from build123d import *

# Parameters (mm, degrees)
F0_W      = 78
F0_H      = 3
F1_DEPTH  = 78
F2_W      = 4
F2_H      = 78
F3_DEPTH  = 28
F4_W      = 4
F4_H      = 78
F5_DEPTH  = 28
F6_W      = 78
F6_H      = 3
F7_DEPTH  = 15
F8_W      = 78
F8_H      = 3
F9_DEPTH  = 15
F12_R     = 3.217192
F13_DEPTH = 22.5
F14_R     = 3.037913
F15_DEPTH = 18.4
F10_R     = 6.245135
F16_DEPTH = 2
F11_R     = 4
F17_DEPTH = 12.6


with BuildPart() as f1:
    # F0 (on Front) → F1 (new body)
    with BuildSketch(Plane.XZ):
        with Locations((4.030592, -1.5)):
            Rectangle(F0_W, F0_H)
    extrude(amount=F1_DEPTH)

    # F2 (on face) → F3 (join)
    with BuildSketch(Plane.XY):
        with Locations((-32.969408, -39)):
            Rectangle(F2_W, F2_H)
    extrude(amount=F3_DEPTH)

    # F4 (on face) → F5 (join)
    with BuildSketch(Plane.XY):
        with Locations((41.030592, -39)):
            Rectangle(F4_W, F4_H)
    extrude(amount=F5_DEPTH)

    # F6 (on face) → F7 (join)
    with BuildSketch(Plane(origin=(-34.969408, 0, 0), x_dir=(0, -1, 0), z_dir=(-1, 0, 0))):
        with Locations((39, 26.5)):
            Rectangle(F6_W, F6_H)
    extrude(amount=F7_DEPTH)

    # F8 (on face) → F9 (join)
    with BuildSketch(Plane.YZ.offset(43.030592)):
        with Locations((-39, 26.5)):
            Rectangle(F8_W, F8_H)
    extrude(amount=F9_DEPTH)

    # F12 (on face) → F13 (cut)
    with BuildSketch(Plane.XY.offset(28)):
        with Locations((47.882639, -9.369526)):
            Circle(F12_R)
        with Locations((47.882639, -68.630474)):
            Circle(F12_R)
    extrude(amount=-F13_DEPTH, mode=Mode.SUBTRACT)

    # F14 (on face) → F15 (cut)
    with BuildSketch(Plane.XY.offset(28)):
        with Locations((-40.469408, -8.328774)):
            Circle(F14_R)
        with Locations((-40.469408, -69.671226)):
            Circle(F14_R)
    extrude(amount=-F15_DEPTH, mode=Mode.SUBTRACT)

    # F10 (on face) → F16 (cut)
    with BuildSketch(Plane.XY):
        with Locations((4.030592, -39)):
            Circle(F10_R)
    extrude(amount=-F16_DEPTH, mode=Mode.SUBTRACT)

    # F11 (on face) → F17 (cut)
    with BuildSketch(Plane.XY):
        with Locations((-24.21356, -9.677462)):
            Circle(F11_R)
        with Locations((32.274744, -9.677462)):
            Circle(F11_R)
        with Locations((-24.21356, -68.322538)):
            Circle(F11_R)
        with Locations((32.274744, -68.322538)):
            Circle(F11_R)
    extrude(amount=-F17_DEPTH, mode=Mode.SUBTRACT)


solid = f1.part
Work out the finished part from the listing and answer in its coordinate system (mm). A direction names the side the tool comes from. Give positions to 0.01 mm unless a question says otherwise; leave off trailing zeros. Loops run counter-clockwise (first coordinate to the right, second up) from the corner with the lowest first, then second, coordinate; pieces in that order, holes last. Notation, with made-up numbers: (12.25, 10.5) - (27.25, 10.5) arc R27 cw to (27.25, 36.5) - close; hole circle Ø11 at (1, 5.5). An arc over 180 degrees is marked (long way). Answer in a Markdown table with one row per item. Add a question column.
Q1. The part is cut by section B-B (y = -39). Determine the outline of the cut face in (x, z), and give its area (3 significant figures).
Q2. A tool of negligible diameter and unlimited length cuts with its end or side. For faces 1 (the flat face through (-42, -38, 25)), 2 (the flat face through (4, -39, -2)), 3 (the flat face through (39.031, -40, 14)), from which of +Z, -Z, +X, -X, +Y, -Y can it reach the whole face along a straight path? Write none if from no direction.
Q3. Determine the mould class of faces 4 (the flat face through (-40, -38, 28)), 5 (the flat face through (3.8, 0, -0.2)), 6 (the cylindrical face through (-27.39, -12.11, -1.48)) for opening direction Y: released by +Y, released by -Y, zero draft, split by the parting line, or undercut.
Q4. The part is cut by section C-C (x = 6). Determine the outline of the cut face in (y, z), and give its area (3 significant figures).
Q5. The part is cut by section A-A (z = 14.5). Determine the outline of the cut face in (x, y), and give its area (3 significant figures).
Q6. The part is cut by section D-D (y = -26.5). Determine the outline of the cut face in (x, z), and give its area (3 significant figures).
Q7. Consider line 1 along X through (y, z) = (-51, 11); line 2 along X through (y, z) = (-20.5, 26); line 3 along Z through (x, y) = (-20, -25). Determine where each line is inside the solid, lowest interval first.
Q8. Each of these flat-tipped pins is pushed along its axis until it touches: P1, Ø6.5, axis at x = -24.21, y = -68.32, coming from the +Z side; P2, Ø14, axis at y = -30.5, z = 13, coming from the -X side; P3, Ø7.5, axis at x = 53.5, y = -32, coming from the -Z side; P4, Ø1, axis at y = -20.5, z = 1.5, coming from the +X side. Where does it stop, or does it pass through?
Solution:
| question | item | result |
|---|---|---|
| 1 | outline | (-49.97, 25) - (-34.97, 25) - (-34.97, -3) - (43.03, -3) - (43.03, 25) - (58.03, 25) - (58.03, 28) - (39.03, 28) - (39.03, 0) - (10.28, 0) - (10.28, -2) - (-2.21, -2) - (-2.21, 0) - (-30.97, 0) - (-30.97, 28) - (-49.97, 28) - close |
| 1 | area | 523 mm² |
| 2 | face 1 | -Z, -X, +Y, -Y |
| 2 | face 2 | +Z |
| 2 | face 3 | +Z, +Y, -Y |
| 3 | face 4 | zero draft |
| 3 | face 5 | released by +Y |
| 3 | face 6 | undercut |
| 4 | outline | (-78, -3) - (0, -3) - (0, 0) - (-33.07, 0) - (-33.07, -2) - (-44.93, -2) - (-44.93, 0) - (-78, 0) - close |
| 4 | area | 210 mm² |
| 5 | outline | (-34.97, -78) - (-30.97, -78) - (-30.97, 0) - (-34.97, 0) - close; (39.03, -78) - (43.03, -78) - (43.03, 0) - (39.03, 0) - close |
| 5 | area | 624 mm² |
| 6 | outline | (-49.97, 25) - (-34.97, 25) - (-34.97, -3) - (43.03, -3) - (43.03, 25) - (58.03, 25) - (58.03, 28) - (39.03, 28) - (39.03, 0) - (-30.97, 0) - (-30.97, 28) - (-49.97, 28) - close |
| 6 | area | 548 mm² |
| 7 | line 1 | x = -34.97 to -30.97, 39.03 to 43.03 |
| 7 | line 2 | x = -49.97 to -30.97, 39.03 to 58.03 |
| 7 | line 3 | z = -3 to 0 |
| 8 | P1 | passes through |
| 8 | P2 | stops at x = -34.97 |
| 8 | P3 | stops at z = 25 |
| 8 | P4 | stops at x = 43.03 |
